Input: part model. Units: mm. Frame: model coordinates. A direction names the side the tool comes from. Coordinates: 2 decimals unless noted, no trailing zeros. Write each loop counter-clockwise with the first axis right and the second up, starting at its lowest first coordinate (ties: lowest second). Pieces come first, ordered by that corner, then holes. Notation, with made-up numbers: (41.25, -29) - (63.25, -29) arc R16 cw to (63.25, -24) - close; hole circle Ø8 at (-24, 83). An arc over 180 degrees is marked (long way). Use CSV: the item, a comma, the result in double quotes.
```python
from build123d import *

# Parameters (mm, degrees)
F0_W     = 70
F0_H     = 120
F1_DEPTH = 60
F2_R     = 2
F3_W     = 34
F3_H     = 40
F3_W_2   = 32
F3_H_2   = 38
F4_DEPTH = 25
F7_W     = 12
F7_H     = 12
F8_DEPTH = 15


with BuildPart() as f1:
    # F0 (on Front) → F1 (new body)
    with BuildSketch(Plane.XZ):
        Rectangle(F0_W, F0_H)
    extrude(amount=F1_DEPTH)

    # F2
    f2_edges = [f1.edges().sort_by_distance(p)[0] for p in [
        (35, -30, 60),
        (35, -30, -60),
        (-35, -30, 60),
        (-35, -30, -60),
        (0, -60, -60),
        (35, -60, 0),
        (0, -60, 60),
        (-35, -60, 0),
    ]]
    fillet(f2_edges, radius=F2_R)

    # F3 (on face) → F4 (cut)
    with BuildSketch(Plane.XZ.offset(60)):
        Rectangle(F3_W, F3_H)
        Rectangle(F3_W_2, F3_H_2, mode=Mode.SUBTRACT)
    extrude(amount=-F4_DEPTH, mode=Mode.SUBTRACT)

    # F7 (on face) → F8 (join, symmetric)
    with BuildSketch(Plane(origin=(0, -55.980762, 15), x_dir=(-1, 0, 0), z_dir=(0, 0.965926, -0.258819))):
        with Locations((0, -15.529143)):
            Rectangle(F7_W, F7_H)
    extrude(amount=F8_DEPTH, both=True)


solid = f1.part
```
(1) Cut plane A-A on x = -8. Return loops of the section in (y, z), and give its area (3 significant figures).
Check values:
outline,"(-60, -58) arc R2 ccw to (-58, -60) - (0, -60) - (0, 60) - (-58, 60) arc R2 ccw to (-60, 58) - (-60, 20) - (-35, 20) - (-35, 19) - (-60, 19) - (-60, -19) - (-35, -19) - (-35, -20) - (-60, -20) - close"
area,"7,150 mm^2"
(2) Reachability of faces 4 (the flat face through (0.08, -66.38, 7.92)), 5 (the flat face through (0, -48, -19)), 6 (the flat face through (-6, -66, 2)), 7 (the flat face through (0, -29, -60)), 8 (the flat face through (6, -66, 2)) from +Z, -Z, +X, -X, +Y, -Y: full face, straight path, thin tool, end or side. Return the list, or none.
Check values:
face 4,"+Z, +X, -X"
face 5,"-Y"
face 6,"+Z, -Z, -X, -Y"
face 7,"-Z, +X, -X, +Y, -Y"
face 8,"+Z, -Z, +X, -Y"
(3) Ray query, probe 1 along Y at (x, z) = (-24.5, 55.5); probe 2 along X at (y, z) = (-58.5, 20.5). Return the intervals inside material, ascending. Write a range as from..to.
Check values:
probe 1,"-60..0"
probe 2,"-34.94..34.94"
(4) Draft query along X for faces 1 (the flat face through (-35, -29, -1)), 2 (the flat face through (0.08, -74.47, 3.96)), 3 (the flat face through (-17, -48, 0)). Return one class per face: pulls with the +X half, pulls with the -X half, needs draft (parallel to the pull), parting line crosses it, or undercut.
Check values:
face 1,"pulls with the -X half"
face 2,"needs draft"
face 3,"undercut"
(5) Cut plane D-D on y = -70. Return loops of the section in (x, z), and give its area (3 significant figures).
Check values:
outline,"(-6, -3.53) - (6, -3.53) - (6, 8.89) - (-6, 8.89) - close"
area,"149 mm^2"
(6) Cut plane C-C on x = 22. Return loops of the section in (y, z).
Check values:
outline,"(-60, -58) arc R2 ccw to (-58, -60) - (0, -60) - (0, 60) - (-58, 60) arc R2 ccw to (-60, 58) - close"
(7) Cut plane B-B on z = 52.5. Return loops of the section in (x, y), and give its area (3 significant figures).
Check values:
outline,"(-35, -58) arc R2 ccw to (-33, -60) - (33, -60) arc R2 ccw to (35, -58) - (35, 0) - (-35, 0) - close"
area,"4,200 mm^2"
(8) Pin query (flat end, axial travel): pin 1 Ø17.5 at (y, z) = (-68, 2) entering from -X; pin 2 Ø8 at (y, z) = (-68, 4.5) entering from +X. Return the tip coordinate at first contact, or that it passes through.
Check values:
pin 1,"x = -34.56"
pin 2,"x = 6"
